Here's the drawing with two shaded views (mm, measured from the low corner). I have some questions. Coordinates: 2 decimals unless noted, no trailing zeros. Write each loop counter-clockwise with the first axis right and the second up, starting at its lowest first coordinate (ties: lowest second). Pieces come first, ordered by that corner, then holes.
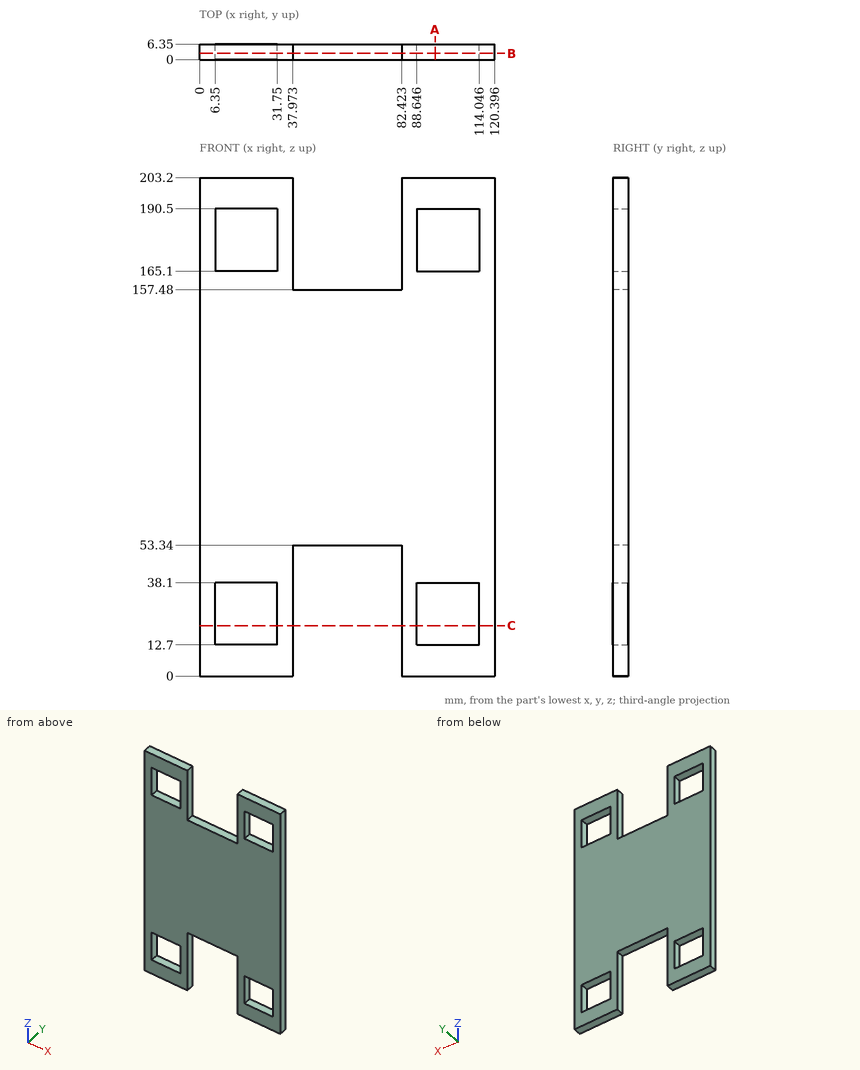
1. If we section it at C-C, the plane z = 20.5: List the corners of the cut face in (x, y) for me, plus the area to 3 significant figures.
2. If we section it at A-A, the plane x = 96: List the corners of the cut face in (y, z) for me.
3. I'm going to push a flat-ended pin straight in: P1, Ø1.5, axis at x = 41, y = 5.5, coming from the +Z side. Where does the tip first touch, or does it pass through?
4. If I drill on L1, parallel to Z at x = 7, y = 1.25; L2, parallel to X at y = 4, z = 193.5; L3, parallel to X at y = 2.5, z = 23, over which ranges is the centre line in solid material (lowest first)?
5. If we section it at B-B, the plane y = 2.5: List the corners of the cut face in (x, z) for me.
Answers:
1. outline: (0, 0) - (6.35, 0) - (6.35, 6.35) - (0, 6.35) - close; (31.75, 0) - (37.97, 0) - (37.97, 6.35) - (31.75, 6.35) - close; (82.42, 0) - (88.65, 0) - (88.65, 6.35) - (82.42, 6.35) - close; (114.05, 0) - (120.4, 0) - (120.4, 6.35) - (114.05, 6.35) - close
1. area: 160 mm2
2. outline: (0, 0) - (6.35, 0) - (6.35, 12.7) - (0, 12.7) - close; (0, 38.1) - (6.35, 38.1) - (6.35, 165.1) - (0, 165.1) - close; (0, 190.5) - (6.35, 190.5) - (6.35, 203.2) - (0, 203.2) - close
3. P1: stops at z = 157.48
4. L1: z = 0 to 12.7, 38.1 to 165.1, 190.5 to 203.2
4. L2: x = 0 to 37.97, 82.42 to 120.4
4. L3: x = 0 to 6.35, 31.75 to 37.97, 82.42 to 88.65, 114.05 to 120.4
5. outline: (0, 0) - (37.97, 0) - (37.97, 53.34) - (82.42, 53.34) - (82.42, 0) - (120.4, 0) - (120.4, 203.2) - (82.42, 203.2) - (82.42, 157.48) - (37.97, 157.48) - (37.97, 203.2) - (0, 203.2) - close; hole (6.35, 12.7) - (31.75, 12.7) - (31.75, 38.1) - (6.35, 38.1) - close; hole (6.35, 165.1) - (31.75, 165.1) - (31.75, 190.5) - (6.35, 190.5) - close; hole (88.65, 12.7) - (114.05, 12.7) - (114.05, 38.1) - (88.65, 38.1) - close; hole (88.65, 165.1) - (114.05, 165.1) - (114.05, 190.5) - (88.65, 190.5) - close
